Verification items for the finished model (mm, model axes). A direction names the side the tool comes from. Round coordinates to 2 decimals unless told otherwise and drop trailing zeros. Order: outer loops, then holes, each group sorted by start corner. A loop starts at its lowest first (then second) coordinate and runs counter-clockwise, first axis right, second up.
```python
from build123d import *

# Parameters (mm, degrees)
SKETCH1_W           = 78.53
SKETCH1_H           = 58.08
SKETCH1_R           = 1.905
SKETCH1_W_2         = 62.491610006
SKETCH1_H_2         = 40.253760829
BOSS_EXTRUDE1_DEPTH = 2.54
CUT_EXTRUDE1_DEPTH  = 2.54


with BuildPart() as part:
    # Sketch1 → Boss-Extrude1 (new body)
    with BuildSketch(Plane(origin=(0, 0, 0), x_dir=(1, 0, 0), z_dir=(0, 1, 0))):
        with Locations((-0.329128556, 0.204655215)):
            Rectangle(SKETCH1_W, SKETCH1_H)
        with Locations(Location((-4.402236218, -22.797237123, 0), (0, 0, 270))):
            Circle(SKETCH1_R, mode=Mode.SUBTRACT)
        with Locations(Location((4.197763782, -22.797237123, 0), (0, 0, 270))):
            Circle(SKETCH1_R, mode=Mode.SUBTRACT)
        with Locations((-0.298250033, 0.894255625)):
            Rectangle(SKETCH1_W_2, SKETCH1_H_2, mode=Mode.SUBTRACT)
    extrude(amount=BOSS_EXTRUDE1_DEPTH)

    # Sketch2 → Cut-Extrude1 (cut)
    with BuildSketch(Plane(origin=(0, 2.54, 0), x_dir=(1, 0, 0), z_dir=(0, 1, 0))):
        with BuildLine():
            Line((-8.568685341, 24.564329148), (7.910428229, 24.564329148))
            ThreePointArc((7.910428229, 24.564329148), (11.453621336, 21.02113604), (7.910428229, 17.477942933))
            Line((7.910428229, 17.477942933), (-8.568685341, 17.477942933))
            ThreePointArc((-8.568685341, 17.477942933), (-12.111878448, 21.02113604), (-8.568685341, 24.564329148))
        make_face()
    extrude(amount=-CUT_EXTRUDE1_DEPTH, mode=Mode.SUBTRACT)


solid = part.part
```
1) Go/stop test with a flat-tipped pin: pin 1 Ø3.5 at (x, z) = (4.2, 22.8) entering from -Y. Record where the tip stops, or that it passes through.
2) Draft check along X on faces 3 (the flat face through (-1, 1, 28.835)), 4 (the flat face through (-39.594, 1, 0)), 5 (the flat face through (38.936, 1, 0)), 6 (the flat face through (-22, 1, -21.021)). Enter one of: released by +X, released by -X, zero draft, split by the parting line, or undercut.
3) Scan lines: probe 1 along Z at (x, y) = (-8.5, 1.05); probe 2 along X at (y, z) = (1.15, 17); probe 3 along Z at (x, y) = (19, 1.9). Record each from-to range of solid material in increasing order.
4) Sectioned sample at B-B on z = 3.5. Record the cut outline in (x, y).
5) Sectioned sample at C-C on y = 1.65. Record the cut outline in (x, z) (3 decimals).
6) Tool access check on faces 1 (the flat face through (-1, 1, 19.233)), 2 (the flat face through (-1, 1, -29.245)). Record the directions out of +Z, -Z, +X, -X, +Y, -Y that give a thin tool (end or side, any length) a straight path to the whole face; none if there is none.
7) Sectioned sample at A-A on x = 0. Record the cut outline in (y, z), then the cut area to 3 significant figures.
Returned:
1. pin 1: passes through
2. face 3: zero draft
2. face 4: released by -X
2. face 5: released by +X
2. face 6: undercut
3. probe 1: z = -29.24 to -24.56, 19.23 to 28.84
3. probe 2: x = -39.59 to -31.54, 30.95 to 38.94
3. probe 3: z = -29.24 to -21.02, 19.23 to 28.84
4. outline: (-39.59, 0) - (-31.54, 0) - (-31.54, 2.54) - (-39.59, 2.54) - close; (30.95, 0) - (38.94, 0) - (38.94, 2.54) - (30.95, 2.54) - close
5. outline: (-39.594, -29.245) - (38.936, -29.245) - (38.936, 28.835) - (-39.594, 28.835) - close; hole (-31.544, -21.021) - (-12.112, -21.021) arc R3.543 ccw to (-8.569, -24.564) - (7.91, -24.564) arc R3.543 ccw to (11.454, -21.021) - (30.948, -21.021) - (30.948, 19.233) - (-31.544, 19.233) - close; hole circle Ø3.81 at (-4.402, 22.797); hole circle Ø3.81 at (4.198, 22.797)
6. face 1: +Y, -Y
6. face 2: -Z, +X, -X, +Y, -Y
7. outline: (0, -29.24) - (2.54, -29.24) - (2.54, -24.56) - (0, -24.56) - close; (0, 19.23) - (2.54, 19.23) - (2.54, 28.84) - (0, 28.84) - close
7. area: 36.3 mm2
